from build123d import *

# Parameters (mm, degrees)
F1_DEPTH = 3
F2_SIZE  = 1
F3_DEPTH = 3.001


with BuildPart() as f1:
    # F0 (on Front) → F1 (new body)
    with BuildSketch(Plane.XZ):
        with BuildLine():
            ThreePointArc((-7.451205, 5.047727), (-2.639996, -8.604093), (9, 0))
            ThreePointArc((9, 0), (8.604093, 2.639996), (7.451205, 5.047727))
            ThreePointArc((7.451205, 5.047727), (0, 4.3), (-7.451205, 5.047727))
        make_face()
        with BuildLine():
            ThreePointArc((-7.451205, 5.047727), (0, 4.3), (7.451205, 5.047727))
            ThreePointArc((7.451205, 5.047727), (0, 9), (-7.451205, 5.047727))
        make_face()
    extrude(amount=-F1_DEPTH)

    # F2
    f2_edges = [f1.edges().sort_by_distance(p)[0] for p in [
        (-9, 0, 0),
    ]]
    chamfer(f2_edges, length=F2_SIZE)

    # F0 (on Front) → F3 (cut, through all)
    with BuildSketch(Plane.XZ):
        with BuildLine():
            ThreePointArc((-7.451205, 5.047727), (0, 4.3), (7.451205, 5.047727))
            ThreePointArc((7.451205, 5.047727), (0, 9), (-7.451205, 5.047727))
        make_face()
    extrude(amount=-F3_DEPTH, mode=Mode.SUBTRACT)


solid = f1.part
Geometry check sheet. Reference: the model listing, model coordinates, mm. Give positions to 0.01 mm unless a question says otherwise; leave off trailing zeros. Loops run counter-clockwise (first coordinate to the right, second up) from the corner with the lowest first, then second, coordinate; pieces in that order, holes last. Notation, with made-up numbers: M 69.25,-11.5 L 77.25,-11.5 A35 ccw 77.25,24.5 Z; hole C 8,30 d7. An arc over 180 degrees is marked long. Answer as a JSON object with one key per item and string values. Group by question number.
Item 1: Mould release check, pull along X, two halves, no side actions. Record for faces 1 (the cylindrical face through (-0.1, 1.5, 4.3)), 2 (the flat face through (0, 3, -2)): pulls with the +X half, pulls with the -X half, needs draft (parallel to the pull), parting line crosses it, or undercut.
Item 2: Material ranges on L1, parallel to Z at x = -7.25, y = 2.9; L2, parallel to Z at x = -6.75, y = 0.45; L3, parallel to X at y = 0.75, z = -4.5, recorded low to high.
Item 3: Gauge pin test, flat ends, axial feed: pin 1 (1.5 mm diameter, centred on y = 2, z = -5.5, fed in from -X); pin 2 (1.5 mm diameter, centred on x = 2, y = 1.5, fed in from -Z); pin 3 (1.5 mm diameter, centred on x = -2, y = 2.5, fed in from +Z). Record the tip position at first contact, or that the pin passes through.
Item 4: Sectioned sample at C-C on y = 0.3. Record the boundary of the cut face in (x, z), plus the area to 3 significant figures.
Item 5: Sectioned sample at B-B on y = 2.3. Record the boundary of the cut face in (x, z), plus the area to 3 significant figures.
Item 6: Sectioned sample at A-A on x = 0. Record the boundary of the cut face in (y, z).
Findings below:
{
 "1": {"face 1": "undercut", "face 2": "needs draft"},
 "2": {"L1": "-5.33 to 5.01", "L2": "-5.08 to 4.91", "L3": "-7.5 to 7.5"},
 "3": {"pin 1": "x = -7.64", "pin 2": "z = -8.91", "pin 3": "z = 4.4"},
 "4": {"outline": "M -6.7,4.9 A8.3 ccw long 8.3,0 A8.3 ccw 6.87,4.66 A8.3 ccw 6.7,4.9 A37.5 cw Z", "area": "179 mm2"},
 "5": {"outline": "M -7.45,5.05 A9 ccw long 9,0 A9 ccw 7.45,5.05 A37.5 cw Z", "area": "206 mm2"},
 "6": {"outline": "M 0,-8 L 1,-9 L 3,-9 L 3,4.3 L 0,4.3 Z"}
}
